Build history of the part. All positions in model axes, mm. A direction names the side the tool comes from. Give positions to 0.01 mm unless a question says otherwise; leave off trailing zeros. Write each loop counter-clockwise with the first axis right and the second up, starting at its lowest first coordinate (ties: lowest second). Pieces come first, ordered by that corner, then holes. Notation, with made-up numbers: (-39.75, 55) -> (7.25, 55) arc R20 cw to (7.25, 84) -> close; hole circle Ø9 at (-9, 14.5). An arc over 180 degrees is marked (long way). Put each result on its own line as item: value.
from build123d import *

# Parameters (mm, degrees)
SKETCH1_W                = 34
SKETCH1_H                = 30
BOSS_EXTRUDE2_DEPTH      = 51
SKETCH3_R                = 2.55
CUT_EXTRUDE3_DEPTH       = 10
SKETCH5_R                = 7.75
CUT_EXTRUDE4_DEPTH       = 51
SKETCH6_W                = 7
SKETCH6_H                = 30
CUT_EXTRUDE6_DEPTH       = 51
CUT_EXTRUDE7_DEPTH       = 51
CUT_EXTRUDE9_DEPTH       = 1.5
CUT_EXTRUDE9_DEPTH_BACK  = 1.5
BOSS_EXTRUDE5_DEPTH      = 51
CUT_EXTRUDE10_DEPTH      = 13
CUT_EXTRUDE11_DEPTH      = 13
SKETCH13_W               = 2
SKETCH13_H               = 6
CUT_EXTRUDE12_DEPTH      = 2
CUT_EXTRUDE13_DEPTH      = 13
CUT_EXTRUDE13_DEPTH_BACK = 11
BOSS_EXTRUDE6_DEPTH      = 2.25
BOSS_EXTRUDE7_DEPTH      = 2.25
BOSS_EXTRUDE8_DEPTH      = 2.25
BOSS_EXTRUDE9_DEPTH      = 2.25
SKETCH22_W               = 5
SKETCH22_H               = 6
BOSS_EXTRUDE10_DEPTH     = 1
SKETCH24_W               = 5
SKETCH24_H               = 6
BOSS_EXTRUDE11_DEPTH     = 1
SKETCH25_R               = 0.6
CUT_EXTRUDE14_DEPTH      = 20
SKETCH26_R               = 2.55
BOSS_EXTRUDE12_DEPTH     = 1.5
CUT_EXTRUDE17_DEPTH      = 60


with BuildPart() as part:
    # Sketch1 → Boss-Extrude2 (new body)
    with BuildSketch(Plane(origin=(0, 0, 0), x_dir=(0, 0, -1), z_dir=(1, 0, 0))):
        with Locations((-3.945183, 6.145902)):
            Rectangle(SKETCH1_W, SKETCH1_H)
    extrude(amount=BOSS_EXTRUDE2_DEPTH)

    # Sketch3 → Cut-Extrude3 (cut)
    with BuildSketch(Plane(origin=(0, 0, -13.054817), x_dir=(-1, 0, 0), z_dir=(0, 0, -1))):
        with Locations((-25.5, -1.354098)):
            Circle(SKETCH3_R)
    extrude(amount=-CUT_EXTRUDE3_DEPTH, mode=Mode.SUBTRACT)

    # Sketch5 → Cut-Extrude4 (cut)
    with BuildSketch(Plane(origin=(51, 0, 0), x_dir=(0, 0, -1), z_dir=(1, 0, 0))):
        with Locations((-3.945183, 1.145902)):
            Circle(SKETCH5_R)
    extrude(amount=-CUT_EXTRUDE4_DEPTH, mode=Mode.SUBTRACT)

    # Sketch6 → Cut-Extrude6 (cut)
    with BuildSketch(Plane(origin=(51, 0, 0), x_dir=(0, 0, -1), z_dir=(1, 0, 0))):
        with Locations((9.554817, 6.145902)):
            Rectangle(SKETCH6_W, SKETCH6_H)
    extrude(amount=-CUT_EXTRUDE6_DEPTH, mode=Mode.SUBTRACT)

    # Sketch7 → Cut-Extrude7 (cut)
    with BuildSketch(Plane(origin=(51, 0, 0), x_dir=(0, 0, -1), z_dir=(1, 0, 0))):
        with BuildLine():
            Line((-3.945183, -8.854098), (-20.945183, -8.854098))
            Line((-20.945183, -8.854098), (-20.945183, 21.145902))
            Line((-20.945183, 21.145902), (6.054817, 21.145902))
            Line((6.054817, 21.145902), (6.054817, 1.145902))
            ThreePointArc((6.054817, 1.145902), (-11.016251, 8.21697), (-3.945183, -8.854098))
        make_face()
    extrude(amount=-CUT_EXTRUDE7_DEPTH, mode=Mode.SUBTRACT)

    # Sketch8 → Cut-Extrude9 (cut, two sides)
    with BuildSketch(Plane(origin=(0, 0, -3.054817), x_dir=(-1, 0, 0), z_dir=(0, 0, -1))) as cut_extrude9_sk:
        Polygon((-21.75, -2.180132), (-21.75, -4.904098), (-29.25, -4.904098), (-29.25, -2.180132), (-29.25, 2.195902), (-21.75, 2.195902), align=None)
    extrude(amount=CUT_EXTRUDE9_DEPTH, mode=Mode.SUBTRACT)
    extrude(cut_extrude9_sk.sketch, amount=-CUT_EXTRUDE9_DEPTH_BACK, mode=Mode.SUBTRACT)

    # Sketch10 → Boss-Extrude5 (add)
    with BuildSketch(Plane(origin=(51, 0, 0), x_dir=(0, 0, -1), z_dir=(1, 0, 0))):
        Polygon((-17.695183, 1.145902), (-17.695183, 4.145902), (-11.695183, 4.145902), (-11.695183, 1.145902), (-11.695183, -1.854098), (-17.695183, -1.854098), align=None)
    extrude(amount=-BOSS_EXTRUDE5_DEPTH)

    # Sketch11 → Cut-Extrude10 (cut)
    with BuildSketch(Plane(origin=(51, 0, 0), x_dir=(0, 0, -1), z_dir=(1, 0, 0))):
        with BuildLine():
            Line((-13.484575, -1.854098), (-17.695183, -1.854098))
            Line((-17.695183, -1.854098), (-17.695183, 4.145902))
            Line((-17.695183, 4.145902), (-13.484575, 4.145902))
            ThreePointArc((-13.484575, 4.145902), (-13.945183, 1.145902), (-13.484575, -1.854098))
        make_face()
    extrude(amount=-CUT_EXTRUDE10_DEPTH, mode=Mode.SUBTRACT)

    # Sketch12 → Cut-Extrude11 (cut)
    with BuildSketch(Plane.ZY):
        with BuildLine():
            Line((13.484575, -1.854098), (17.695183, -1.854098))
            Line((17.695183, -1.854098), (17.695183, 4.145902))
            Line((17.695183, 4.145902), (13.484575, 4.145902))
            ThreePointArc((13.484575, 4.145902), (13.945183, 1.145902), (13.484575, -1.854098))
        make_face()
    extrude(amount=-CUT_EXTRUDE11_DEPTH, mode=Mode.SUBTRACT)

    # Sketch13 → Cut-Extrude12 (cut)
    with BuildSketch(Plane.XY.offset(17.695183)):
        with Locations((25.5, 1.145902)):
            Rectangle(SKETCH13_W, SKETCH13_H)
    extrude(amount=-CUT_EXTRUDE12_DEPTH, mode=Mode.SUBTRACT)

    # Sketch15 → Cut-Extrude13 (cut, two sides)
    with BuildSketch(Plane(origin=(24.5, 0, 0), x_dir=(0, 0, -1), z_dir=(1, 0, 0))) as cut_extrude13_sk:
        with BuildLine():
            Line((-17.695183, 4.145902), (-17.695183, -1.854098))
            Line((-17.695183, -1.854098), (-13.484575, -1.854098))
            ThreePointArc((-13.484575, -1.854098), (-13.945183, 1.145902), (-13.484575, 4.145902))
            Line((-13.484575, 4.145902), (-17.695183, 4.145902))
        make_face()
    extrude(amount=CUT_EXTRUDE13_DEPTH, mode=Mode.SUBTRACT)
    extrude(cut_extrude13_sk.sketch, amount=-CUT_EXTRUDE13_DEPTH_BACK, mode=Mode.SUBTRACT)

    # Sketch17 → Boss-Extrude6 (add)
    with BuildSketch(Plane(origin=(38, 0, 0), x_dir=(0, 0, -1), z_dir=(1, 0, 0))):
        with BuildLine():
            Line((-13.484575, 4.145902), (-17.695183, 4.145902))
            Line((-17.695183, 4.145902), (-17.695183, -1.854098))
            Line((-17.695183, -1.854098), (-13.484575, -1.854098))
            ThreePointArc((-13.484575, -1.854098), (-13.945183, 1.145902), (-13.484575, 4.145902))
        make_face()
    extrude(amount=BOSS_EXTRUDE6_DEPTH)

    # Sketch19 → Boss-Extrude7 (add)
    with BuildSketch(Plane.ZY.offset(-13)):
        with BuildLine():
            Line((13.484575, 4.145902), (17.695183, 4.145902))
            Line((17.695183, 4.145902), (17.695183, -1.854098))
            Line((17.695183, -1.854098), (13.484575, -1.854098))
            ThreePointArc((13.484575, -1.854098), (13.945183, 1.145902), (13.484575, 4.145902))
        make_face()
    extrude(amount=BOSS_EXTRUDE7_DEPTH)

    # Sketch20 → Boss-Extrude8 (add)
    with BuildSketch(Plane(origin=(13.5, 0, 0), x_dir=(0, 0, -1), z_dir=(1, 0, 0))):
        with BuildLine():
            Line((-17.695183, -1.854098), (-17.695183, 4.145902))
            Line((-17.695183, 4.145902), (-13.484575, 4.145902))
            ThreePointArc((-13.484575, 4.145902), (-13.945183, 1.145902), (-13.484575, -1.854098))
            Line((-13.484575, -1.854098), (-17.695183, -1.854098))
        make_face()
    extrude(amount=BOSS_EXTRUDE8_DEPTH)

    # Sketch21 → Boss-Extrude9 (add)
    with BuildSketch(Plane.ZY.offset(-37.5)):
        with BuildLine():
            Line((13.484575, 4.145902), (17.695183, 4.145902))
            Line((17.695183, 4.145902), (17.695183, -1.854098))
            Line((17.695183, -1.854098), (13.484575, -1.854098))
            ThreePointArc((13.484575, -1.854098), (13.945183, 1.145902), (13.484575, 4.145902))
        make_face()
    extrude(amount=BOSS_EXTRUDE9_DEPTH)

    # Sketch22 → Boss-Extrude10 (add)
    with BuildSketch(Plane.XY.offset(17.695183)):
        with Locations((37.75, 1.145902)):
            Rectangle(SKETCH22_W, SKETCH22_H)
    extrude(amount=BOSS_EXTRUDE10_DEPTH)

    # Sketch24 → Boss-Extrude11 (add)
    with BuildSketch(Plane.XY.offset(17.695183)):
        with Locations((13.25, 1.145902)):
            Rectangle(SKETCH24_W, SKETCH24_H)
    extrude(amount=BOSS_EXTRUDE11_DEPTH)

    # Sketch25 → Cut-Extrude14 (cut)
    with BuildSketch(Plane(origin=(0, 4.145902, 0), x_dir=(1, 0, 0), z_dir=(0, 1, 0))):
        with Locations((13.25, -16.695183)):
            Circle(SKETCH25_R)
        with Locations((37.75, -16.695183)):
            Circle(SKETCH25_R)
    extrude(amount=-CUT_EXTRUDE14_DEPTH, mode=Mode.SUBTRACT)

    # Sketch26 → Boss-Extrude12 (add)
    with BuildSketch(Plane(origin=(0, 0, -6.054817), x_dir=(-1, 0, 0), z_dir=(0, 0, -1))):
        with Locations((-25.5, -1.354098)):
            Circle(SKETCH26_R)
    extrude(amount=-BOSS_EXTRUDE12_DEPTH)

    # Sketch27 → Cut-Extrude17 (cut)
    with BuildSketch(Plane(origin=(51, 0, 0), x_dir=(0, 0, -1), z_dir=(1, 0, 0))):
        Polygon((-18.695183, 1.145902), (-18.695183, 1.645902), (6.594767, 1.645902), (6.594767, 1.145902), (6.594767, 0.645902), (6.594767, -9.845584), (-18.695183, -9.845584), (-18.695183, 0.645902), align=None)
    extrude(amount=-CUT_EXTRUDE17_DEPTH, mode=Mode.SUBTRACT)


solid = part.part
1) Slice it at A-A (x = 37.75). Write the cut outline in (y, z), plus the area to 3 significant figures.
Filled sheet:
outline: (1.65, -6.04) arc R10 ccw to (4.15, 13.48) -> (4.15, 16.1) -> (1.65, 16.1) -> (1.65, 11.68) arc R7.75 cw to (1.65, -3.79) -> close; (1.65, 17.3) -> (4.15, 17.3) -> (4.15, 18.7) -> (1.65, 18.7) -> close
area: 69.8 mm2
2) Pin check, flat tips, straight feed: pin 1 (1 mm diameter, centred on x = 42.5, y = 9, fed in from +Z); pin 2 (2 mm diameter, centred on y = 3.5, z = 16.5, fed in from +X); pin 3 (1.5 mm diameter, centred on x = 26.5, y = 7, fed in from +Z); pin 4 (3 mm diameter, centred on y = 5, z = 14.5, fed in from -X). Stop position of each tip, or through.
Filled sheet:
pin 1: z = 10.72
pin 2: x = 40.25
pin 3: z = 12.54
pin 4: x = 0
3) Slice it at D-D (y = 7.25). Write the cut outline in (x, z), plus the area to 3 significant figures.
Filled sheet:
outline: (0, -3.98) -> (51, -3.98) -> (51, -0.83) -> (0, -0.83) -> close; (0, 8.72) -> (51, 8.72) -> (51, 11.87) -> (0, 11.87) -> close
area: 321 mm2
4) Slice it at B-B (y = 2.75). Write the cut outline in (x, z), plus the area to 3 significant figures.
Filled sheet:
outline: (0, -5.93) -> (51, -5.93) -> (51, -3.64) -> (0, -3.64) -> close; (0, 11.53) -> (51, 11.53) -> (51, 13.82) -> (40.25, 13.82) -> (40.25, 18.7) -> (35.25, 18.7) -> (35.25, 13.82) -> (15.75, 13.82) -> (15.75, 18.7) -> (10.75, 18.7) -> (10.75, 13.82) -> (0, 13.82) -> close; hole circle Ø1.2 at (13.25, 16.7); hole circle Ø1.2 at (37.75, 16.7)
area: 280 mm2
5) Slice it at C-C (x = 28). Write the cut outline in (y, z).
Filled sheet:
outline: (1.65, -6.04) arc R10 ccw to (1.65, 13.93) -> (1.65, 11.68) arc R7.75 cw to (2.2, -3.73) -> (2.2, -4.55) -> (1.65, -4.55) -> close
6) Tool access for faces 5 (the flat face through (38, 4.146, 15)), 6 (the flat face through (13, 3, 18.695)): list every direction of +Z, -Z, +X, -X, +Y, -Y with a clear straight run to the whole face (end or side of a thin tool).
Filled sheet:
face 5: +Z, +X, -X, +Y
face 6: +Z, +X, -X, +Y, -Y
7) Wall check: L1, parallel to Z at x = 37.75, y = 3.65; L2, parallel to Z at x = 37.75, y = 2.3; L3, parallel to Z at x = 46, y = 4.5. Give the ranges that are in metal, low to high.
Filled sheet:
L1: -5.74 to -3.39, 11.28 to 16.1, 17.3 to 18.7
L2: -5.99 to -3.72, 11.61 to 16.1, 17.3 to 18.7
L3: -5.48 to -3.04, 10.93 to 13.37
8) Pull direction Z, two halves, no side cores. Call faces 1 (the cylindrical face through (13.17, 2.91, 16.1)), 2 (the flat face through (51, 9.2, 3.9)), 3 (the flat face through (38, 3, 18.695)), 4 (the cylindrical face through (38.07, 2.91, 16.19)): released by +Z, released by -Z, zero draft, split by the parting line, or undercut.
Filled sheet:
face 1: undercut
face 2: zero draft
face 3: released by +Z
face 4: undercut
